Check sheet for the modelled part. Datum: model origin and axes. Units: mm. A direction names the side the tool comes from. Round coordinates to 2 decimals unless told otherwise and drop trailing zeros. Loops run counter-clockwise (first coordinate to the right, second up) from the corner with the lowest first, then second, coordinate; pieces in that order, holes last. Notation, with made-up numbers: (24, -2) - (67, -2) arc R14 cw to (67, 19) - close; hole circle Ø4 at (38.5, 12). An arc over 180 degrees is marked (long way). Put each result on its own line as item: value. Start each with the question number.
Item 1: Gauge pin test, flat end, axial feed: pin 1 Ø5.5 at (x, y) = (-12.7, 0) entering from +Z. Record the tip position at first contact, or that the pin passes through.
Item 2: Section check A-A, the plane y = 0. Record the cut outline in (x, z).
Item 3: Tool access check on faces 1 (the cylindrical face through (10.47, -0.92, 1)), 2 (the cylindrical face through (8.956, 3.433, 2.547)). Record the directions out of +Z, -Z, +X, -X, +Y, -Y that give a thin tool (end or side, any length) a straight path to the whole face; none if there is none.
Item 4: Section check C-C, the plane z = 0.9. Record the cut outline in (x, y), and give its area (3 significant figures).
Item 5: Material ranges on line 1 along X through (y, z) = (-4, 2.1); line 2 along X through (y, z) = (2, 0.2); line 3 along Y through (x, z) = (-12.7, 2.5), recorded low to high.
Item 6: Section check B-B, the plane x = -12.7. Record the cut outline in (y, z), and give its area (3 significant figures).
Item 7: Section check D-D, the plane x = 13. Record the cut outline in (y, z), and give its area (3 significant figures).
Item 8: Draft check along Y on faces 3 (the flat face through (0, -12.7, 2)), 4 (the cylindrical face through (-16.73, -3.09, 2.55)), 5 (the flat face through (0, 0, 3.048)). Enter one of: pulls with the +Y half, pulls with the -Y half, needs draft (parallel to the pull), parting line crosses it, or undercut.
from build123d import *

# Parameters (mm, degrees)
SKETCH_W         = 50.8
SKETCH_H         = 25.4
PAD_DEPTH        = 3.048
HOLE_D           = 4.826
HOLE_DEPTH       = 635
HOLE_CBORE_D     = 10.16
HOLE_CBORE_DEPTH = 1.016


with BuildPart() as part:
    # Sketch → Pad (new body)
    with BuildSketch(Plane.XY):
        Rectangle(SKETCH_W, SKETCH_H)
    extrude(amount=PAD_DEPTH)

    # Hole
    with Locations(Plane.XY.offset(3.048)):
        with Locations((-12.7, 0), (12.7, 0)):
            CounterBoreHole(HOLE_D / 2, HOLE_CBORE_D / 2, HOLE_CBORE_DEPTH, depth=HOLE_DEPTH)


solid = part.part
Check result:
1. pin 1: z = 2.03
2. outline: (-25.4, 0) - (-15.11, 0) - (-15.11, 2.03) - (-17.78, 2.03) - (-17.78, 3.05) - (-25.4, 3.05) - close; (-10.29, 0) - (10.29, 0) - (10.29, 2.03) - (7.62, 2.03) - (7.62, 3.05) - (-7.62, 3.05) - (-7.62, 2.03) - (-10.29, 2.03) - close; (15.11, 0) - (25.4, 0) - (25.4, 3.05) - (17.78, 3.05) - (17.78, 2.03) - (15.11, 2.03) - close
3. face 1: +Z, -Z
3. face 2: +Z
4. outline: (-25.4, -12.7) - (25.4, -12.7) - (25.4, 12.7) - (-25.4, 12.7) - close; hole circle Ø4.83 at (-12.7, 0); hole circle Ø4.83 at (12.7, 0)
4. area: 1,250 mm²
5. line 1: -25.4 to -15.83, -9.57 to 9.57, 15.83 to 25.4
5. line 2: -25.4 to -14.05, -11.35 to 11.35, 14.05 to 25.4
5. line 3: -12.7 to -5.08, 5.08 to 12.7
6. outline: (-12.7, 0) - (-2.41, 0) - (-2.41, 2.03) - (-5.08, 2.03) - (-5.08, 3.05) - (-12.7, 3.05) - close; (2.41, 0) - (12.7, 0) - (12.7, 3.05) - (5.08, 3.05) - (5.08, 2.03) - (2.41, 2.03) - close
6. area: 57.3 mm²
7. outline: (-12.7, 0) - (-2.39, 0) - (-2.39, 2.03) - (-5.07, 2.03) - (-5.07, 3.05) - (-12.7, 3.05) - close; (2.39, 0) - (12.7, 0) - (12.7, 3.05) - (5.07, 3.05) - (5.07, 2.03) - (2.39, 2.03) - close
7. area: 57.4 mm²
8. face 3: pulls with the -Y half
8. face 4: undercut
8. face 5: needs draft
